Read the model definition and answer for the solid it produces. Units are mm, in the model's axes. Face numbers are marked on the shaded views. A direction names the side the tool comes from. Give positions to 0.01 mm unless a question says otherwise; leave off trailing zeros. Order: outer loops, then holes, each group sorted by start corner. A loop starts at its lowest first (then second) coordinate and runs counter-clockwise, first axis right, second up. Notation, with made-up numbers: (80, -31) - (137, -31) arc R15 cw to (137, -12) - close; hole circle Ø7 at (8, 44.5). An arc over 180 degrees is marked (long way). Write each question's results on one line, items separated by ' | '.
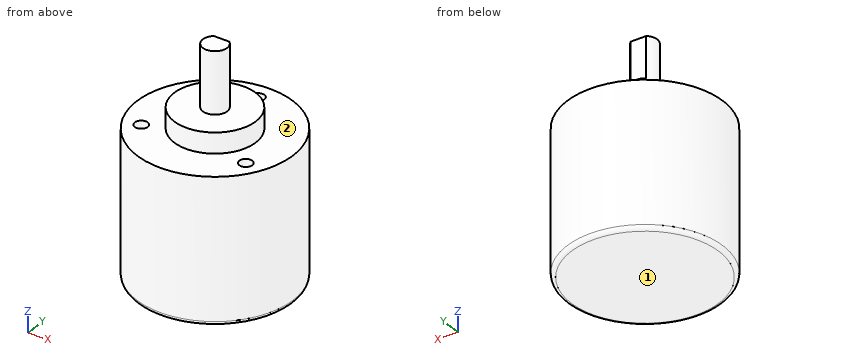
from build123d import *

# Parameters (mm, degrees)
SKETCH_1_R          = 19.1
EXTRUDE_1_DEPTH     = 35.2
SKETCH_2_R          = 10
EXTRUDE_2_DEPTH     = 5
SKETCH_4_R          = 1.6
CUT_EXTRUDE_1_DEPTH = 5
SKETCH_5_R          = 3
EXTRUDE_3_DEPTH     = 15
CUT_EXTRUDE_START   = -10
CUT_EXTRUDE_2_DEPTH = 10
FILLET_1_R          = 1


with BuildPart() as part:
    # 草图1 → 凸台-拉伸1 (new body)
    with BuildSketch(Plane.XY):
        Circle(SKETCH_1_R)
    extrude(amount=EXTRUDE_1_DEPTH)

    # 草图2 → 凸台-拉伸2 (add)
    with BuildSketch(Plane.XY.offset(35.2)):
        Circle(SKETCH_2_R)
    extrude(amount=EXTRUDE_2_DEPTH)

    # 草图4 → 切除-拉伸1 (cut)
    with BuildSketch(Plane.XY.offset(35.2)):
        with Locations((0, 15)):
            Circle(SKETCH_4_R)
        with Locations((12.990381057, -7.5)):
            Circle(SKETCH_4_R)
        with Locations((-12.990381057, -7.5)):
            Circle(SKETCH_4_R)
    extrude(amount=-CUT_EXTRUDE_1_DEPTH, mode=Mode.SUBTRACT)

    # 草图5 → 凸台-拉伸3 (add)
    with BuildSketch(Plane.XY.offset(40.2)):
        Circle(SKETCH_5_R)
    extrude(amount=EXTRUDE_3_DEPTH)

    # 草图6 → 切除-拉伸2 (cut)
    with BuildSketch(Plane.XY.offset(55.2).offset(CUT_EXTRUDE_START)):
        with BuildLine():
            Line((-1.926136028, 2.3), (1.926136028, 2.3))
            ThreePointArc((1.926136028, 2.3), (0, 3), (-1.926136028, 2.3))
        make_face()
    extrude(amount=CUT_EXTRUDE_2_DEPTH, mode=Mode.SUBTRACT)

    # 圆角1
    fillet_1_edges = [part.edges().sort_by_distance(p)[0] for p in [
        (-19.1, 0, 0),
    ]]
    fillet(fillet_1_edges, radius=FILLET_1_R)


solid = part.part
(1) For the marked faces 1 and 2, determine the directions among +Z, -Z, +X, -X, +Y, -Y from which every point of the face is accessible in a straight line to the end or side of a thin tool.
Conclusion:
face 1: -Z, +X, -X, +Y, -Y | face 2: +Z
(2) Section D-D (z = 50) is taken. Give the vertices of the cut face in (x, y).
Conclusion:
outline: (-1.93, 2.3) arc R3 ccw (long way) to (1.93, 2.3) - close
(3) Each of these flat-tipped pins is pushed along its axis until it touches: pin 1 (4 mm diameter, centred on x = -14, z = 28.5, fed in from +Y); pin 2 (11.5 mm diameter, centred on x = -2.5, y = 3.5, fed in from +Z); pin 3 (1 mm diameter, centred on x = -13.5, y = -7, fed in from +Z); pin 4 (3.5 mm diameter, centred on x = -12.99, y = -7.5, fed in from +Z). Where does it stop, or does it pass through?
Conclusion:
pin 1: y = 14.86 | pin 2: z = 55.2 | pin 3: z = 30.2 | pin 4: z = 35.2
(4) Section A-A (x = 0) is taken. Give the vertices of the cut face in (y, z).
Conclusion:
outline: (-19.1, 1) arc R1 ccw to (-18.1, 0) - (18.1, 0) arc R1 ccw to (19.1, 1) - (19.1, 35.2) - (16.6, 35.2) - (16.6, 30.2) - (13.4, 30.2) - (13.4, 35.2) - (10, 35.2) - (10, 40.2) - (3, 40.2) - (3, 45.2) - (2.3, 45.2) - (2.3, 55.2) - (-3, 55.2) - (-3, 40.2) - (-10, 40.2) - (-10, 35.2) - (-19.1, 35.2) - close
(5) Consider probe 1 along Y at (x, z) = (0, 33); probe 2 along X at (y, z) = (-7, 33); probe 3 along Z at (x, y) = (15, -3). Determine where each line is inside the solid, lowest interval first. Write a range as [from, to].
Conclusion:
probe 1: [-19.1, 13.4], [16.6, 19.1] | probe 2: [-17.77, -14.51], [-11.47, 11.47], [14.51, 17.77] | probe 3: [0, 35.2]
(6) Section B-B (y = 0) is taken. Give the vertices of the cut face in (x, z), plus the area to 3 significant figures.
Conclusion:
outline: (-19.1, 1) arc R1 ccw to (-18.1, 0) - (18.1, 0) arc R1 ccw to (19.1, 1) - (19.1, 35.2) - (10, 35.2) - (10, 40.2) - (3, 40.2) - (3, 55.2) - (-3, 55.2) - (-3, 40.2) - (-10, 40.2) - (-10, 35.2) - (-19.1, 35.2) - close | area: 1,530 mm^2
(7) Section C-C (z = 38.5) is taken. Give the vertices of the cut face in (x, y).
Conclusion:
outline: circle Ø20 at (0, 0)
